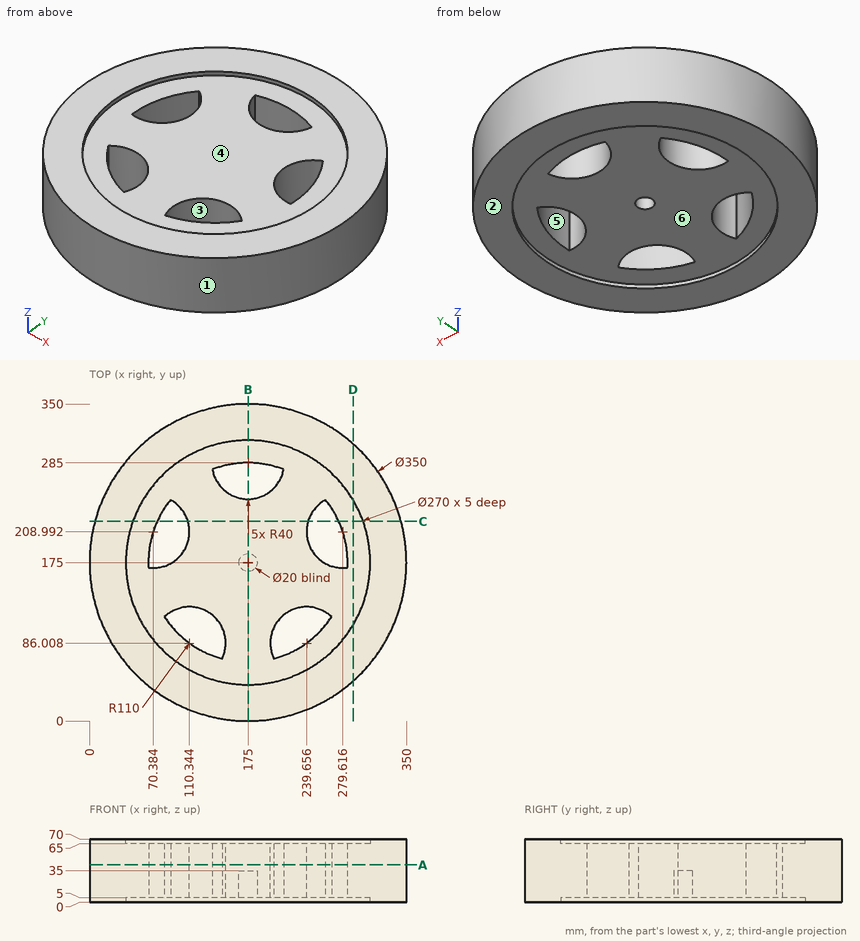
Can you work these out from the drawing? Everything is in mm from the part's minimum corner. A direction names the side the tool comes from. Round coordinates to 2 decimals unless told otherwise and drop trailing zeros. Order: outer loops, then holes, each group sorted by start corner. A loop starts at its lowest first (then second) coordinate and runs counter-clockwise, first axis right, second up. Notation, with made-up numbers: (54, -35.5) -> (60, -35.5) arc R22 ccw to (60, -16.5) -> close; hole circle Ø4 at (-11.5, -28.75). An arc over 180 degrees is marked (long way). Return JSON: item names as keys, results as strings. Group by question number.
1. If we section it at B-B, the plane x = 175: Write out the boundary of the cut face in (y, z).
2. If we section it at D-D, the plane x = 291: Write out the boundary of the cut face in (y, z), then the cut area to 3 significant figures.
3. We'd pull the mould along Y, two halves only. Please class the marked faces 1, 2 and 3: released by +Y, released by -Y, zero draft, split by the parting line, or undercut.
4. If we section it at C-C, the plane y = 220.5: Write out the boundary of the cut face in (x, z).
5. Will these pins go through, and if not, where does the flat tip stop? pin 1 (4 mm diameter, centred on x = 146, z = 22, fed in from -Y) (1 decimal); pin 2 (1.5 mm diameter, centred on x = 190.5, y = 49.5, fed in from +Z); pin 3 (1.5 mm diameter, centred on x = 44, z = 17.5, fed in from +Y) (1 decimal).
6. Which directions (+Z, -Z, +X, -X, +Y, -Y) give clear straight access to the entire face, cutting with the end or side of a thin tool? Please do the marked faces 4, 5 and 6.
7. I need wall thicknesses on line 1 (Y direction, x = 175, z = 2.05); line 2 (Y direction, x = 168.5, z = 33.5); line 3 (Z direction, x = 134.5, y = 176). Which ranges of each line are inside material? Lowest first, please. Write a range as [from, to].
8. If we section it at A-A, the plane z = 41.5: Write out the boundary of the cut face in (x, y) (1 decimal).
Output values:
{
 "1": {"outline": "(0, 0) -> (40, 0) -> (40, 5) -> (165, 5) -> (165, 35) -> (185, 35) -> (185, 5) -> (245, 5) -> (245, 65) -> (40, 65) -> (40, 70) -> (0, 70) -> close; (285, 5) -> (310, 5) -> (310, 0) -> (350, 0) -> (350, 70) -> (310, 70) -> (310, 65) -> (285, 65) -> close"},
 "2": {"outline": "(43.97, 0) -> (105.94, 0) -> (105.94, 5) -> (244.06, 5) -> (244.06, 0) -> (306.03, 0) -> (306.03, 70) -> (244.06, 70) -> (244.06, 65) -> (105.94, 65) -> (105.94, 70) -> (43.97, 70) -> close", "area": "17,000 mm²"},
 "3": {"face 1": "split by the parting line", "face 2": "zero draft", "face 3": "undercut"},
 "4": {"outline": "(6.02, 0) -> (47.9, 0) -> (47.9, 5) -> (74.85, 5) -> (74.85, 65) -> (47.9, 65) -> (47.9, 70) -> (6.02, 70) -> close; (108.69, 5) -> (241.31, 5) -> (241.31, 65) -> (108.69, 65) -> close; (275.15, 5) -> (302.1, 5) -> (302.1, 0) -> (343.98, 0) -> (343.98, 70) -> (302.1, 70) -> (302.1, 65) -> (275.15, 65) -> close"},
 "5": {"pin 1": "y = 2.1", "pin 2": "z = 65", "pin 3": "y = 291.9"},
 "6": {"face 4": "+Z", "face 5": "+Z, -Z", "face 6": "-Z"},
 "7": {"line 1": "[0, 40], [310, 350]", "line 2": "[0.12, 167.4], [182.6, 245.53], [284.81, 349.88]", "line 3": "[5, 65]"},
 "8": {"outline": "circle Ø350 at (175, 175); hole (65.1, 169.3) arc R40 ccw to (89.5, 244.2) arc R110 ccw to start; hole (82.8, 115) arc R110 ccw to (146.4, 68.8) arc R40 ccw to start; hole (135.7, 277.7) arc R40 ccw to (214.3, 277.7) arc R110 ccw to start; hole (203.6, 68.8) arc R110 ccw to (267.2, 115) arc R40 ccw to start; hole (260.5, 244.2) arc R40 ccw to (284.9, 169.3) arc R110 ccw to start"}
}
